Could you check a few things on this model? Use its own coordinates, in mm. Coordinates: 2 decimals unless noted, no trailing zeros. Order: outer loops, then holes, each group sorted by start corner. A loop starts at its lowest first (then second) coordinate and runs counter-clockwise, first axis right, second up.
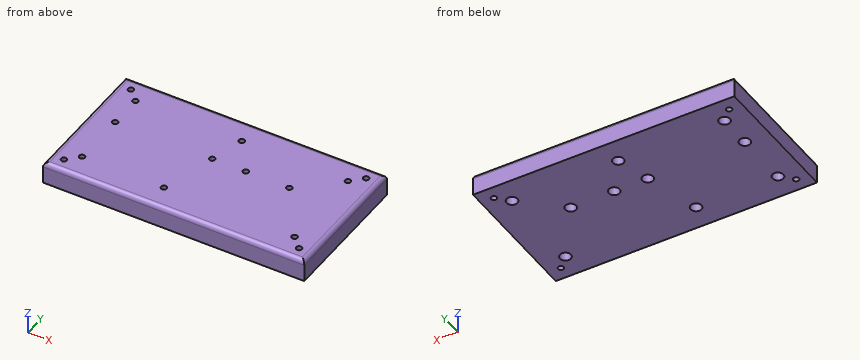
```python
from build123d import *

# Parameters (mm, degrees)
F0_W     = 300
F0_H     = 158
F1_DEPTH = 25
F2_R     = 5
F3_R     = 3.25
F4_DEPTH = 25
F5_R     = 3.25
F6_DEPTH = 25
F7_R     = 6.25
F8_DEPTH = 15


with BuildPart() as f1:
    # F0 (on Top) → F1 (new body)
    with BuildSketch(Plane.XY):
        with Locations((150, 79)):
            Rectangle(F0_W, F0_H)
    extrude(amount=F1_DEPTH)

    # F2
    f2_edges = [f1.edges().sort_by_distance(p)[0] for p in [
        (0, 79, 25),
        (150, 158, 25),
        (150, 0, 25),
        (300, 79, 25),
    ]]
    fillet(f2_edges, radius=F2_R)

    # F3 (on face) → F4 (cut)
    with BuildSketch(Plane(origin=(0, 0, 0), x_dir=(1, 0, 0), z_dir=(0, 0, -1))):
        with Locations((15, -15)):
            Circle(F3_R)
        with Locations((285, -15)):
            Circle(F3_R)
        with Locations((15, -143)):
            Circle(F3_R)
        with Locations((285, -143)):
            Circle(F3_R)
    extrude(amount=-F4_DEPTH, mode=Mode.SUBTRACT)

    # F5 (on face) → F6 (cut)
    with BuildSketch(Plane(origin=(0, 0, 0), x_dir=(1, 0, 0), z_dir=(0, 0, -1))):
        with Locations((272, -28)):
            Circle(F5_R)
        with Locations((28, -28)):
            Circle(F5_R)
        with Locations((28, -130)):
            Circle(F5_R)
        with Locations((272, -130)):
            Circle(F5_R)
        with Locations((150, -130)):
            Circle(F5_R)
        with Locations((122, -28)):
            Circle(F5_R)
        with Locations((28, -91.2)):
            Circle(F5_R)
        with Locations((139.5, -91.2)):
            Circle(F5_R)
        with Locations((178, -91.2)):
            Circle(F5_R)
        with Locations((228, -91.2)):
            Circle(F5_R)
    extrude(amount=-F6_DEPTH, mode=Mode.SUBTRACT)

    # F7 (on face) → F8 (cut)
    with BuildSketch(Plane(origin=(0, 0, 0), x_dir=(1, 0, 0), z_dir=(0, 0, -1))):
        with Locations((28, -28)):
            Circle(F7_R)
        with Locations((122, -28)):
            Circle(F7_R)
        with Locations((272, -28)):
            Circle(F7_R)
        with Locations((228, -91.2)):
            Circle(F7_R)
        with Locations((178, -91.2)):
            Circle(F7_R)
        with Locations((139.5, -91.2)):
            Circle(F7_R)
        with Locations((150, -130)):
            Circle(F7_R)
        with Locations((272, -130)):
            Circle(F7_R)
        with Locations((28, -130)):
            Circle(F7_R)
        with Locations((28, -91.2)):
            Circle(F7_R)
    extrude(amount=-F8_DEPTH, mode=Mode.SUBTRACT)


solid = f1.part
```
Item 1: Suppose I cut it at D-D (z = 8.5). Count the separate pieces of the cut face and the enclosed holes in it, and give its area (3 significant figures).
Item 2: Suppose I cut it at C-C (x = 285). List the corners of the cut face in (y, z) for me, and give its area (3 significant figures).
Item 3: I need wall thicknesses on line 1 (X direction, y = 130, z = 17.75); line 2 (X direction, y = 91.2, z = 19.5); line 3 (Y direction, x = 28, z = 5.75). Which ranges of each line are inside material? Lowest first, please.
Item 4: Suppose I cut it at B-B (x = 228). List the corners of the cut face in (y, z) for me.
Item 5: Suppose I cut it at A-A (y = 143). List the corners of the cut face in (x, z) for me, and give its area (3 significant figures).
Item 6: For pin 1 Ø6 at (x, y) = (139.5, 91.2) entering from -Z; pin 2 Ø8.5 at (x, y) = (150, 130) entering from -Z, each with a flat end and sliding along its axis, tell me the tip position at first contact or that it passes through.
Geometry results:
1. separate pieces: 1
1. enclosed holes: 14
1. area: 46,000 mm2
2. outline: (0, 0) - (11.75, 0) - (11.75, 25) - (5, 25) arc R5 ccw to (0, 20) - close; (18.25, 0) - (139.75, 0) - (139.75, 25) - (18.25, 25) - close; (146.25, 0) - (158, 0) - (158, 20) arc R5 ccw to (153, 25) - (146.25, 25) - close
2. area: 3,610 mm2
3. line 1: x = 0 to 24.75, 31.25 to 146.75, 153.25 to 268.75, 275.25 to 300
3. line 2: x = 0 to 24.75, 31.25 to 136.25, 142.75 to 174.75, 181.25 to 224.75, 231.25 to 300
3. line 3: y = 0 to 21.75, 34.25 to 84.95, 97.45 to 123.75, 136.25 to 158
4. outline: (0, 0) - (84.95, 0) - (84.95, 15) - (87.95, 15) - (87.95, 25) - (5, 25) arc R5 ccw to (0, 20) - close; (94.45, 15) - (97.45, 15) - (97.45, 0) - (158, 0) - (158, 20) arc R5 ccw to (153, 25) - (94.45, 25) - close
5. outline: (0, 0) - (11.75, 0) - (11.75, 25) - (5, 25) arc R5 ccw to (0, 20) - close; (18.25, 0) - (281.75, 0) - (281.75, 25) - (18.25, 25) - close; (288.25, 0) - (300, 0) - (300, 20) arc R5 ccw to (295, 25) - (288.25, 25) - close
5. area: 7,160 mm2
6. pin 1: passes through
6. pin 2: stops at z = 15
